Geometry check sheet. Reference: the model listing, model coordinates, mm. Face numbers are marked on the shaded views. A direction names the side the tool comes from. Give positions to 0.01 mm unless a question says otherwise; leave off trailing zeros. Loops run counter-clockwise (first coordinate to the right, second up) from the corner with the lowest first, then second, coordinate; pieces in that order, holes last. Notation, with made-up numbers: (6.25, 37) -> (34.25, 37) arc R24 cw to (34.25, 64) -> close; hole circle Ø7 at (-10, 15). An arc over 180 degrees is marked (long way). Write item = value, one per line.
Autodesk Inventor part; units mm, degrees
ref_plane "Work Plane2" through (0, 0, 0) normal (0, 0, 1) x (1, 0, 0)
ref_plane "YZ Plane" through (0, 0, 0) normal (1, 0, 0) x (0, 1, 0)
ref_plane "XZ Plane" through (0, 0, 0) normal (0, 1, 0) x (-1, 0, 0)
ref_plane "Work Plane1" through (22.2, 37.1, 6) normal (0, 0, -1) x (0, 1, 0)
ref_plane "Work Plane2" through (0, 0, 0) normal (0, 0, 1) x (1, 0, 0)
sketch "Sketch1" plane through (22.2, 37.1, 6) normal (0, 0, -1) x (0, 1, 0)
  circle A0 centre (25.9, 3.8) radius 1.75
  circle A1 centre (25.9, -16.2) radius 1.75
  circle A2 centre (5.9, 3.8) radius 1.75
  circle A3 centre (5.9, -16.2) radius 1.5
  line L0 (3, -22.4) -> (9.5, -22.4) construction
  line L1 (9.5, 10) -> (9.5, -22.4) construction
  line L2 (3, 10) -> (9.5, 10) construction
  line L3 (3, 10) -> (3, -22.4) construction
  circle A4 centre (5.9, 3.8) radius 1.75 construction
  circle A5 centre (5.9, -16.2) radius 1.75 construction
  line L4 (28.8, -22.4) -> (21.9, -22.4) construction
  line L5 (21.9, 10) -> (21.9, -22.4) construction
  line L6 (28.8, 10) -> (21.9, 10) construction
  line L7 (28.8, 10) -> (28.8, -22.4) construction
  line L8 (19.9, 3.8) -> (19.9, -14.6723) construction
  line L9 (28.8, 10) -> (-33.8945, 10)
  line L10 (-33.8945, 10) -> (-33.8945, -22.4)
  line L11 (-33.8945, -22.4) -> (28.8, -22.4)
  line L12 (28.8, -22.4) -> (28.8, 10)
  line L13 (-33.8945, -22.4) -> (28.8, -22.4)
  line L14 (28.8, -22.4) -> (28.8, -37.4)
  line L15 (28.8, -37.4) -> (-33.8945, -37.4)
  line L16 (-33.8945, -37.4) -> (-33.8945, -22.4)
  line L17 (28.8, 10) -> (-33.8945, 10)
  line L18 (-33.8945, 10) -> (-33.8945, 25)
  line L19 (-33.8945, 25) -> (28.8, 25)
  line L20 (28.8, 25) -> (28.8, 10)
  line L21 (28.8, 25) -> (-33.8945, 10)
  point P0 (-37.1, -22.2)
  point P1 (28.8, -22.4)
extrude "Extrusion1" add sketch "Sketch1" along normal up to surface (6 mm away) contours A0 | A1 | A2 | A3 | L12 L11 L10 L9 | L9 L21 L20 | L18 L19 L21
sketch "Sketch2" plane through (22.2, 37.1, 6) normal (0, 0, 1) x (1, 0, 0)
  line L0 (10, 28.8) -> (10, -33.8945)
  circle A0 centre (-6.2, -29.1) radius 1.4
  line L1 (-6.2, -54.7229) -> (-6.2, -13.0662) construction
  line L2 (10, -33.8945) -> (-22.4, -33.8945)
  line L3 (-4.7, -54.7229) -> (-4.7, -13.0662)
  line L4 (-7.7, -13.0662) -> (-7.7, -54.7229)
  arc A1 (-7.7, -54.7229) -> (-4.7, -54.7229) centre (-6.2, -54.7229) ccw
  arc A2 (-4.7, -13.0662) -> (-7.7, -13.0662) centre (-6.2, -13.0662) ccw
  line L5 (10, -33.8945) -> (-37.4, -33.8945)
  line L6 (-37.4, 28.8) -> (10, 28.8)
  line L7 (-37.4, -33.8945) -> (-37.4, 28.8)
  point P0 (-22.2, -37.1)
  point P1 (-6.2, -33.8945)
  dimension "d2" = 3
extrude "Extrusion2" cut sketch "Sketch2" against normal blind 10 contours L3 A1 L4 L2 | L2 L4 A2 L3 | A0
sketch "Sketch3" plane through (32.2, 65.9, 0) normal (0, 0, -1) x (-1, 0, 0)
  circle A0 centre (6.2, -22.9) radius 1.25
  circle A1 centre (26.2, -22.9) radius 1.25
  circle A2 centre (26.2, -2.9) radius 1.25
  circle A3 centre (6.2, -2.9) radius 1.25
  line L0 (47.4, 0) -> (0, 0)
  point P0 (32.2, -65.9)
  point P1 (14.2, -22.9)
  point P2 (34.2, -22.9)
  point P3 (34.2, -2.9)
  point P4 (14.2, -2.9)
  point P5 (22.2, -22.9)
  point P6 (42.2, -22.9)
  point P7 (42.2, -2.9)
  point P8 (22.2, -2.9)
  dimension "d22" = 8
hole "Hole1" at (6, 63, 0) at (26, 63, 0) at (26, 43, 0) at (6, 43, 0) at (-10, 43, 0) at (-2, 43, 0) at (-2, 63, 0) at (-10, 63, 0) direction (0, 0, 1) diameter 2.9 end through all counterbore diameter 6.5 counterbore depth 4
ref_plane "Work Plane3" through (0.2759, 57, -15.7452) normal (0, -1, 0) x (-0.9087, 0, 0.4175)
sketch "Sketch4" plane through (32.2, 3.2055, 0) normal (0, 0, -1) x (-1, 0, 0)
  line L0 (41.88, 53.7945) -> (-24.48, 53.7945)
  line L1 (32.4, 0) -> (32.4, 37.0885)
  line L2 (0, 62.6945) -> (0, 0)
  line L3 (32.4, 53.7945) -> (0, 53.7945)
  line L4 (0, 53.7945) -> (0, 49.2945)
  line L5 (0, 49.2945) -> (32.4, 49.2945)
  line L6 (32.4, 49.2945) -> (32.4, 53.7945)
  line L7 (32.4, 62.6945) -> (-15, 62.6945)
  line L8 (32.4, 62.6945) -> (0, 62.6945)
  line L9 (0, 62.6945) -> (0, 57.6945)
  line L10 (0, 57.6945) -> (32.4, 57.6945)
  line L11 (32.4, 57.6945) -> (32.4, 62.6945)
  point P0 (32.2, -3.2055)
  point P1 (26.2, 47.7945)
  point P2 (32.4, 49.2945)
  point P3 (0, 53.7945)
  point P4 (0, 53.7945)
  dimension "d12" = 4.5
  dimension "d31" = 5
pattern_linear "Rechteckige Anordnung1" count 3 spacing 8 along (1, 0, 0) of "Hole1"
extrude "Extrusion3" add sketch "Sketch4" along normal blind 28.7 and the other way blind 5 contours L2 L7 L11 L10
sketch "Sketch5" plane through (-0.2, 65.9, 0) normal (0, 1, 0) x (1, 0, 0)
  circle A0 centre (-1.3, 26) radius 1
  circle A1 centre (26.7, 21) radius 1 construction
  circle A2 centre (5.2, 5.5) radius 1 construction
  circle A3 centre (16.2, 16) radius 2.6486
  line L0 (24.5969, 9.4163) -> (7.8031, 9.4163)
  line L1 (7.8031, 9.4163) -> (7.8031, 22.5837)
  line L2 (7.8031, 22.5837) -> (24.5969, 22.5837)
  line L3 (24.5969, 22.5837) -> (24.5969, 9.4163)
  line L4 (24.5969, 9.4163) -> (7.8031, 22.5837) construction
  line L5 (7.8031, 9.4163) -> (24.5969, 22.5837) construction
  circle A4 centre (26.7, 21) radius 0.75
  circle A5 centre (5.2, 5.5) radius 0.75
  point P0 (0.2, 0)
  dimension "d15" = 1.5
  dimension "d16" = 1.5
extrude "Extrusion4" cut sketch "Sketch5" against normal blind 10 contours A3 | L0 L1 L2 L3 | A4 | A5
properties part number "30_cellSTORM_UC2_Laser_holder"
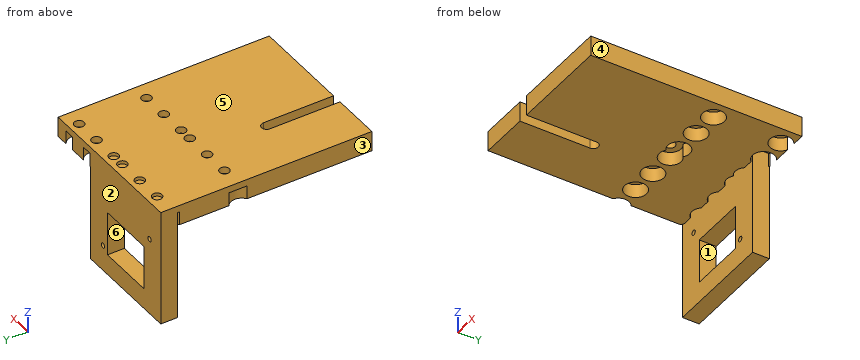
Item 1: Section check B-B, the plane x = 34. Record the cut outline in (y, z), plus the area to 3 significant figures.
Answer:
outline = (3.21, 0) -> (39.75, 0) -> (39.75, 4) -> (41.55, 4) -> (41.55, 6) -> (3.21, 6) -> close; (44.45, 4) -> (46.25, 4) -> (46.25, 0) -> (59.75, 0) -> (59.75, 4) -> (61.55, 4) -> (61.55, 6) -> (44.45, 6) -> close; (64.45, 4) -> (65.9, 4) -> (65.9, 6) -> (64.45, 6) -> close
area = 314 mm^2
Item 2: Gauge pin test, flat ends, axial feed: pin 1 (5.5 mm diameter, centred on y = 63, z = -18.5, fed in from +X); pin 2 (7 mm diameter, centred on x = 41, y = 43, fed in from -Z); pin 3 (1.4 mm diameter, centred on x = 22, y = 63, fed in from +Z). Record the tip position at first contact, or that the pin passes through.
Answer:
pin_1 = 32.2
pin_2 = 0
pin_3 = 5
Item 3: Draft check along X on the marked faces 1, 2, 3 and 4. Enter one of: +X half, -X half, draft (parallel to the pull), parting line (faces both ways), or undercut.
Answer:
face_1 = undercut
face_2 = draft
face_3 = -X half
face_4 = +X half
Item 4: Thickness scan on L1, parallel to Y at x = 42, z = 4.8; L2, parallel to X at y = 63.6, z = -21; L3, parallel to X at y = 43, z = 1.3. Record the ranges inside material, lowest first. Write a range as [from, to].
Answer:
L1 = [3.21, 41.55], [44.45, 61.55], [64.45, 65.9]
L2 = [-0.2, 7.6], [24.4, 25.75], [27.25, 32.2]
L3 = [1.25, 2.75], [9.25, 10.75], [17.25, 18.75], [29.25, 30.75], [37.25, 38.75], [45.25, 47.2]
Item 5: Section check D-D, the plane y = 63. Give the number of separate pieces and of enclosed holes in the cut face, plus the area to 3 significant figures.
Answer:
separate_pieces = 3
enclosed_holes = 3
area = 920 mm^2
Item 6: Section check C-C, the plane z = -21. Record the cut outline in (x, y), plus the area to 3 significant figures.
Answer:
outline = (-0.2, 60.9) -> (7.6, 60.9) -> (7.6, 65.9) -> (-0.2, 65.9) -> close; (24.4, 60.9) -> (25.75, 60.9) -> (25.75, 65.9) -> (24.4, 65.9) -> close; (27.25, 60.9) -> (32.2, 60.9) -> (32.2, 65.9) -> (27.25, 65.9) -> close
area = 70.5 mm^2
Item 7: Tool access check on the marked faces 5 and 6. Record the directions out of +Z, -Z, +X, -X, +Y, -Y that give a thin tool (end or side, any length) a straight path to the whole face; none if there is none.
Answer:
face_5 = +Z, +X, -X, +Y, -Y
face_6 = +Y, -Y
Item 8: Section check A-A, the plane y = 21. Record the cut outline in (x, z).
Answer:
outline = (-0.2, 0) -> (14.5, 0) -> (14.5, 6) -> (-0.2, 6) -> close; (17.5, 0) -> (47.2, 0) -> (47.2, 6) -> (17.5, 6) -> close
